```python
from build123d import *

# Parameters (mm, degrees)
F1_DEPTH = 5


with BuildPart() as f1:
    # F0 (on Front) → F1 (new body)
    with BuildSketch(Plane.XZ):
        with BuildLine():
            ThreePointArc((-6.797868, 4.217699), (2.192835, 7.693599), (8, 0))
            ThreePointArc((8, 0), (5.176145, -6.099797), (-1.301882, -7.893358))
            Line((-1.301882, -7.893358), (55.644045, -17.285668))
            ThreePointArc((55.644045, -17.285668), (51.257847, -3.766855), (64.824389, -8.003125))
            Line((64.824389, -8.003125), (50.932535, 70.781496))
            ThreePointArc((50.932535, 70.781496), (51.02363, 70.089556), (51.054073, 69.39231))
            ThreePointArc((51.054073, 69.39231), (40.861237, 61.698711), (36.256205, 73.61001))
            Line((36.256205, 73.61001), (-6.797868, 4.217699))
        make_face()
        with BuildLine():
            ThreePointArc((-1.301882, -7.893358), (5.176145, -6.099797), (8, 0))
            ThreePointArc((8, 0), (2.192835, 7.693599), (-6.797868, 4.217699))
            ThreePointArc((-6.797868, 4.217699), (-7.284979, -3.305916), (-1.301882, -7.893358))
        make_face()
        with BuildLine():
            ThreePointArc((64.824389, -8.003125), (51.257847, -3.766855), (55.644045, -17.285668))
            ThreePointArc((55.644045, -17.285668), (62.122072, -15.492107), (64.945927, -9.39231))
            ThreePointArc((64.945927, -9.39231), (64.915485, -8.695064), (64.824389, -8.003125))
        make_face()
        with BuildLine():
            ThreePointArc((50.932535, 70.781496), (44.568023, 77.247751), (36.256205, 73.61001))
            ThreePointArc((36.256205, 73.61001), (40.861237, 61.698711), (51.054073, 69.39231))
            ThreePointArc((51.054073, 69.39231), (51.02363, 70.089556), (50.932535, 70.781496))
        make_face()
    extrude(amount=F1_DEPTH)


solid = f1.part
```
CAD build for the part. Positions are in the model's coordinates, mm. Round coordinates to 2 decimals unless told otherwise and drop trailing zeros. Order: outer loops, then holes, each group sorted by start corner. A loop starts at its lowest first (then second) coordinate and runs counter-clockwise, first axis right, second up. Notation, with made-up numbers: (49.25, 62) -> (57.25, 62) arc R12 cw to (57.25, 69) -> close; hole circle Ø5 at (46, 72.5). An arc over 180 degrees is marked (long way). Write item = value, one per line.
(1) Cut at B-B (z = 69). Write the cut outline in (x, y).
Answers follow:
outline = (33.4, -5) -> (51.25, -5) -> (51.25, 0) -> (33.4, 0) -> close
(2) Flat gauge pins, fed straight in: P1, Ø1.5, axis at x = 5.5, y = -3.5, coming from the +Z side; P2, Ø3, axis at y = -4.5, z = 5.5, coming from the -X side; P3, Ø2, axis at y = -2, z = 50, coming from the -X side. Where does each tip first touch, or does it go through?
Answers follow:
P1 = 25.25
P2 = -6.93
P3 = 20.99
(3) Cut at C-C (x = 12). Write the cut outline in (y, z), plus the area to 3 significant figures.
Answers follow:
outline = (-5, -10.09) -> (0, -10.09) -> (0, 34.52) -> (-5, 34.52) -> close
area = 223 mm²
(4) Cut at A-A (y = -4.05). Write the cut outline in (x, z).
Answers follow:
outline = (-6.8, 4.22) arc R8 ccw to (-1.3, -7.89) -> (55.64, -17.29) arc R8 ccw to (64.95, -9.39) arc R8 ccw to (64.82, -8) -> (50.93, 70.78) arc R8 ccw to (36.26, 73.61) -> close
(5) Drill centre lines: L1, parallel to X at y = -1.05, z = 45.5; L2, parallel to X at y = -3.5, z = 65; L3, parallel to Z at x = 22, y = -1.4. Where is each one in solid material? Low to high.
Answers follow:
L1 = 18.82 to 55.39
L2 = 30.91 to 51.95
L3 = -11.74 to 50.63
